```python
from build123d import *

# Parameters (mm, degrees)
F0_W     = 20
F0_H     = 15
F1_DEPTH = 3
F2_W     = 15.5
F2_H     = 6
F3_DEPTH = 25
F4_SIZE2 = 1.5
F4_SIZE  = 2.25


with BuildPart() as f1:
    # F0 (on Top) → F1 (new body)
    with BuildSketch(Plane.XY):
        Rectangle(F0_W, F0_H)
    extrude(amount=F1_DEPTH)

    # F2 (on face) → F3 (cut)
    with BuildSketch(Plane.XY.offset(3)):
        Rectangle(F2_W, F2_H)
    extrude(amount=-F3_DEPTH, mode=Mode.SUBTRACT)

    # F4
    f4_edges = [f1.edges().sort_by_distance(p)[0] for p in [
        (-7.75, 3, 1.5),
        (7.75, 3, 1.5),
    ]]
    f4_side = f1.faces().sort_by_distance((0, 3, 1.5))[0]
    chamfer(f4_edges, length=F4_SIZE, length2=F4_SIZE2, reference=f4_side)


solid = f1.part
```
Read the model definition and answer for the solid it produces. Units are mm, in the model's axes. A direction names the side the tool comes from. Round coordinates to 2 decimals unless told otherwise and drop trailing zeros. Write each loop counter-clockwise with the first axis right and the second up, starting at its lowest first coordinate (ties: lowest second). Pieces come first, ordered by that corner, then holes. Notation, with made-up numbers: M 17,85 L 74,85 A14 cw 74,108 Z; hole C -29.75,71 d8. An arc over 180 degrees is marked long. One line per item, written item: value.
Q1. Which of the six approach directions +Z, -Z, +X, -X, +Y, -Y give full straight-line access (tool end or side, diameter ignored) to faces 4 (the flat face through (7, 2, 2)), 5 (the flat face through (10, 0, 1))?
Data:
face 4: +Z, -Z
face 5: +Z, -Z, +X, +Y, -Y
Q2. Straight lines are drawn through the part: line 1 (Y direction, x = 2.5, z = 1.1); line 2 (X direction, y = 1, z = 0.8); line 3 (Y direction, x = 6, z = 2.85). For each, find the intervals that lie inside material, in ascending order. Write a range as [from, to].
Data:
line 1: [-7.5, -3], [3, 7.5]
line 2: [-10, -7.75], [7.75, 10]
line 3: [-7.5, -3], [2.67, 7.5]
Q3. Find section A-A on x = -7. Write down the section's boundary in (y, z), plus the area to 3 significant figures.
Data:
outline: M -7.5,0 L -3,0 L -3,3 L -7.5,3 Z; M 2,0 L 7.5,0 L 7.5,3 L 2,3 Z
area: 30.0 mm2
Q4. Find section C-C on z = 1.7. Write down the section's boundary in (x, y), plus the area to 3 significant figures.
Data:
outline: M -10,-7.5 L 10,-7.5 L 10,7.5 L -10,7.5 Z; hole M -7.75,-3 L 7.75,-3 L 7.75,1.5 L 5.5,3 L -5.5,3 L -7.75,1.5 Z
area: 210 mm2
Q5. A flat-ended cylindrical pin translates along its axis: pin 1 Ø3 at (x, y) = (7, 2.5) entering from -Z. Find the tip coordinate at first contact, or state that the pin passes through.
Data:
pin 1: z = 0
Q6. For a pull along X with two mould halves and no side action, classify faces 1 (the flat face through (-10, 0, 1)), 2 (the flat face through (0, 3, 2)), 3 (the flat face through (0, 7.5, 1)) as +X half, -X half, draft (parallel to the pull), parting line (faces both ways), or undercut.
Data:
face 1: -X half
face 2: undercut
face 3: draft
Q7. Find section B-B on y = -2.25. Write down the section's boundary in (x, z).
Data:
outline: M -10,0 L -7.75,0 L -7.75,3 L -10,3 Z; M 7.75,0 L 10,0 L 10,3 L 7.75,3 Z
